The model under review builds one solid part; all positions refer to its coordinate system, in mm. A direction names the side the tool comes from. Round coordinates to 2 decimals unless told otherwise and drop trailing zeros. Order: outer loops, then holes, each group sorted by start corner. A loop starts at its lowest first (then second) coordinate and runs counter-clockwise, first axis right, second up. Notation, with made-up numbers: (-23.5, 78) -> (24.5, 78) arc R20 ccw to (24.5, 94) -> close; hole circle Ø8 at (-20.5, 84.5). An arc over 180 degrees is marked (long way). Use a Markdown table: item, result. Add a question column.
```python
from build123d import *

# Parameters (mm, degrees)
F0_R     = 12.7
F1_DEPTH = 793.75
F2_R     = 12.7
F2_R_2   = 9.398
F3_DEPTH = 19.05
F4_R     = 12.7
F4_R_2   = 9.398
F5_DEPTH = 19.05
F6_R     = 9.398
F6_R_2   = 6.35
F7_DEPTH = 12.7
F8_R     = 9.398
F8_R_2   = 6.35
F9_DEPTH = 12.7


with BuildPart() as f1:
    # F0 (on Front) → F1 (new body, symmetric)
    with BuildSketch(Plane.XZ):
        Circle(F0_R)
    extrude(amount=F1_DEPTH, both=True)

    # F2 (on face) → F3 (cut)
    with BuildSketch(Plane(origin=(0, 793.75, 0), x_dir=(-1, 0, 0), z_dir=(0, 1, 0))):
        Circle(F2_R)
        Circle(F2_R_2, mode=Mode.SUBTRACT)
    extrude(amount=-F3_DEPTH, mode=Mode.SUBTRACT)

    # F4 (on face) → F5 (cut)
    with BuildSketch(Plane.XZ.offset(793.75)):
        Circle(F4_R)
        Circle(F4_R_2, mode=Mode.SUBTRACT)
    extrude(amount=-F5_DEPTH, mode=Mode.SUBTRACT)

    # F6 (on face) → F7 (cut)
    with BuildSketch(Plane.XZ.offset(793.75)):
        Circle(F6_R)
        Circle(F6_R_2, mode=Mode.SUBTRACT)
    extrude(amount=-F7_DEPTH, mode=Mode.SUBTRACT)

    # F8 (on face) → F9 (cut)
    with BuildSketch(Plane(origin=(0, 793.75, 0), x_dir=(-1, 0, 0), z_dir=(0, 1, 0))):
        Circle(F8_R)
        Circle(F8_R_2, mode=Mode.SUBTRACT)
    extrude(amount=-F9_DEPTH, mode=Mode.SUBTRACT)


solid = f1.part
```
Q1. Add section B-B, the plane y = 692. Give the boundary of the cut face in (x, z), then the cut area to 3 significant figures.
Q2. To check wall thickness, follow line 1 along Z through (x, y) = (-2.75, 576.5); line 2 along Y through (x, z) = (-2.5, -11); line 3 along Z through (x, y) = (-8.25, -239). State the ranges of each line that lie inside material, in increasing order.
Q3. For faces 1 (the face through (1.8, -774.7, 9.5)), 2 (the face through (-2.75, -10.85, -12.4)), 3 (the face through (-1.8, 774.7, 9.5)), list the 3-axis set-ups (+Z, -Z, +X, -X, +Y, -Y) from which the entire face can be reached by the end or side of a thin tool; tool diameter is ignored.
Q4. For pin 1 (2 mm diameter, centred on x = 6.5, z = -3.5, fed in from +Y); pin 2 (3 mm diameter, centred on y = -471.5, z = 5.5, fed in from -X); pin 3 (12 mm diameter, centred on x = 9, y = 244.5, fed in from +Z), all flat-tipped, find the tip position at first contact; note any pin that passes through.
Q5. Add section A-A, the plane x = -2.25. Give the boundary of the cut face in (y, z).
Return value:
| question | item | result |
|---|---|---|
| 1 | outline | circle Ø25.4 at (0, 0) |
| 1 | area | 507 mm² |
| 2 | line 1 | -12.4 to 12.4 |
| 2 | line 2 | -774.7 to 774.7 |
| 2 | line 3 | -9.66 to 9.66 |
| 3 | face 1 | -Y |
| 3 | face 2 | +Y, -Y |
| 3 | face 3 | +Y |
| 4 | pin 1 | y = 781.05 |
| 4 | pin 2 | x = -12.05 |
| 4 | pin 3 | z = 12.34 |
| 5 | outline | (-793.75, -5.94) -> (-781.05, -5.94) -> (-781.05, -9.12) -> (-774.7, -9.12) -> (-774.7, -12.5) -> (774.7, -12.5) -> (774.7, -9.12) -> (781.05, -9.12) -> (781.05, -5.94) -> (793.75, -5.94) -> (793.75, 5.94) -> (781.05, 5.94) -> (781.05, 9.12) -> (774.7, 9.12) -> (774.7, 12.5) -> (-774.7, 12.5) -> (-774.7, 9.12) -> (-781.05, 9.12) -> (-781.05, 5.94) -> (-793.75, 5.94) -> close |
